```python
from build123d import *

# Parameters (mm, degrees)
F1_DEPTH = 45
F2_R     = 375
F3_DEPTH = 25
F4_R     = 375
F4_R_2   = 275
F5_DEPTH = 140


with BuildPart() as f1:
    # F0 (on Top) → F1 (new body)
    with BuildSketch(Plane.XY):
        Polygon((500, 430), (430, 500), (-430, 500), (-500, 430), (-500, -430), (-430, -500), (430, -500), (500, -430), align=None)
    extrude(amount=F1_DEPTH)

    # F2 (on face) → F3 (join)
    with BuildSketch(Plane.XY.offset(45)):
        with Locations((0, -8.12363)):
            Circle(F2_R)
    extrude(amount=F3_DEPTH)

    # F4 (on face) → F5 (join)
    with BuildSketch(Plane.XY.offset(70)):
        with Locations((0, -8.12363)):
            Circle(F4_R)
        Circle(F4_R_2, mode=Mode.SUBTRACT)
    extrude(amount=F5_DEPTH)


solid = f1.part
```
Model file for the job. Use its own axes, mm. A direction names the side the tool comes from. Round coordinates to 2 decimals unless told otherwise and drop trailing zeros. Write each loop counter-clockwise with the first axis right and the second up, starting at its lowest first coordinate (ties: lowest second). Pieces come first, ordered by that corner, then holes. Notation, with made-up numbers: (57, -4.5) - (91, -4.5) arc R17 cw to (91, 19.5) - close; hole circle Ø6 at (-13, 12). An arc over 180 degrees is marked (long way). One line per item, written item: value.
(1) 3-axis set-ups, long thin cutter, end or side, ignore diameter. For faces 4 (the flat face through (-465, 465, 22)), 5 (the flat face through (-340, 229, 45)): which of +Z, -Z, +X, -X, +Y, -Y reach the whole face in a straight line?
Values follow:
face 4: +Z, -Z, -X, +Y
face 5: +Z
(2) Cut at C-C, the plane z = 190. Give the cut face in (x, y), plus the area to 3 significant figures.
Values follow:
outline: circle Ø750 at (0, -8.12); hole circle Ø550 at (0, 0)
area: 204,000 mm²
(3) Two-plate mould, pull along X, no slides. Class faces 1 (the flat face through (-465, -465, 22)), 2 (the flat face through (465, -465, 22)), 3 (the cylindrical face through (262.3, 82.6, 139)): pulls with the +X half, pulls with the -X half, needs draft (parallel to the pull), parting line crosses it, or undercut.
Values follow:
face 1: pulls with the -X half
face 2: pulls with the +X half
face 3: undercut
(4) Cut at B-B, the plane y = -27. Give the cut face in (x, z).
Values follow:
outline: (-500, 0) - (500, 0) - (500, 45) - (374.52, 45) - (374.52, 210) - (273.67, 210) - (273.67, 70) - (-273.67, 70) - (-273.67, 210) - (-374.52, 210) - (-374.52, 45) - (-500, 45) - close
(5) Cut at A-A, the plane x = 0. Give the cut face in (y, z), plus the area to 4 significant figures.
Values follow:
outline: (-500, 0) - (500, 0) - (500, 45) - (366.88, 45) - (366.88, 210) - (275, 210) - (275, 70) - (-275, 70) - (-275, 210) - (-383.12, 210) - (-383.12, 45) - (-500, 45) - close
area: 91,750 mm²
(6) Wall check: probe 1 along Y at (x, z) = (-10.5, 121); probe 2 along Y at (x, z) = (0, 177); probe 3 along Z at (x, y) = (-93.5, 35.5). Give the ranges that are in metal, low to high.
Values follow:
probe 1: y = -382.98 to -274.8, 274.8 to 366.73
probe 2: y = -383.12 to -275, 275 to 366.88
probe 3: z = 0 to 70
(7) Drop flat-ended pins along their axis: P1, Ø10, axis at x = -139.5, y = 98, coming from the +Z side; P2, Ø12, axis at x = 158, z = 91, coming from the +Y side; P3, Ø1, axis at y = 190.5, z = 53.5, coming from the -X side. Give the stop position or say it passes through.
Values follow:
P1: stops at z = 70
P2: stops at y = 334.69
P3: stops at x = -318.39
(8) Cut at D-D, the plane x = 291. Give the cut face in (y, z).
Values follow:
outline: (-500, 0) - (500, 0) - (500, 45) - (228.4, 45) - (228.4, 210) - (-244.65, 210) - (-244.65, 45) - (-500, 45) - close
